Print and shaded views of the part. All mm, measured from the part's lowest x, y and z. A direction names the side the tool comes from. Round coordinates to 2 decimals unless told otherwise and drop trailing zeros. Order: outer loops, then holes, each group sorted by start corner. A loop starts at its lowest first (then second) coordinate and runs counter-clockwise, first axis right, second up. Notation, with made-up numbers: (11.25, 7) - (40.25, 7) arc R9 ccw to (40.25, 21) - close; hole circle Ø6 at (77, -12.5). An arc over 180 degrees is marked (long way). Write item = value, one per line. Start each with the question number.
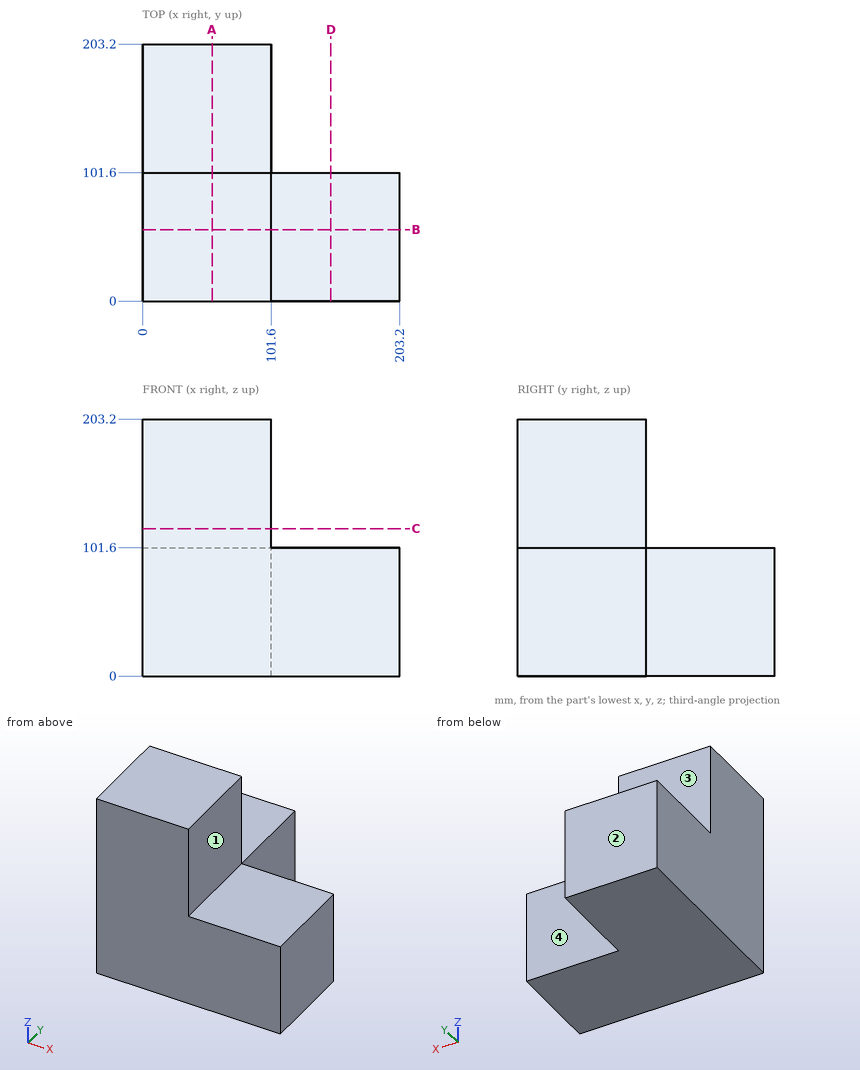
Item 1: Probe L1, parallel to Y at x = 11, z = 139.5. List the from-to ranges inside material, lowest first.
Item 2: Saw through at C-C, the plane z = 116.5. Give the cut face in (x, y).
Item 3: Drop a flat-ended pin along its axis: pin 1 (12 mm diameter, centred on x = 59.5, z = 162.5, fed in from +Y). Give the stop position or say it passes through.
Item 4: Saw through at A-A, the plane x = 55. Give the cut face in (y, z).
Item 5: Which spindle directions (+Z, -Z, +X, -X, +Y, -Y) get a long thin tool onto all of the face, cutting with end or side? Do the marked faces 1, 2, 3 and 4. Say none if no direction does.
Check sheet entries:
q1.L1 = 0 to 101.6
q2.outline = (0, 0) - (101.6, 0) - (101.6, 101.6) - (0, 101.6) - close
q3.pin_1 = 101.6
q4.outline = (0, 0) - (203.2, 0) - (203.2, 101.6) - (101.6, 101.6) - (101.6, 203.2) - (0, 203.2) - close
q5.face_1 = +Z, +X, +Y, -Y
q5.face_2 = +Z, -Z, +X, -X, +Y
q5.face_3 = +Z, +X, -X, +Y
q5.face_4 = +Z, -Z, +X, +Y
